Part model, mm, in its own coordinate system. A direction names the side the tool comes from. Round coordinates to 2 decimals unless told otherwise and drop trailing zeros. Write each loop counter-clockwise with the first axis right and the second up, starting at its lowest first coordinate (ties: lowest second). Pieces come first, ordered by that corner, then holes. Notation, with made-up numbers: M 45,35.5 L 87,35.5 A19 ccw 87,59.5 Z; hole C 44,-20 d9. An arc over 180 degrees is marked long. Use a Markdown table: item, result. Add a question column.
1) Which spindle directions (+Z, -Z, +X, -X, +Y, -Y) get a long thin tool onto all of the face, cutting with end or side? Do faces 1 (the face through (72.697, -22.893, 17.517)), 2 (the face through (-50.3, 15.4, 155.245)). Say none if no direction does.
2) Slice it at A-A on z = 73. Write the cut outline in (x, y), plus the area to 3 significant figures.
3) Wall check: probe 1 along X at (y, z) = (0, 77); probe 2 along Z at (x, y) = (-29, -63.5). Give the ranges that are in metal, low to high.
4) Drop flat-ended pins along their axis: P1, Ø8, axis at x = 22, y = 6.5, coming from the +Z side; P2, Ø4, axis at x = -3, z = 56, coming from the -Y side; P3, Ø10, axis at x = 4.5, z = 87.5, coming from the +Y side. Give the stop position or say it passes through.
5) Two-plate mould, pull along Z, no slides. Class faces 3 (the face through (-37.002, 28.372, 70.543)), 4 (the face through (35, -18, 0)), 5 (the face through (36.432, 70.045, 128.311)): released by +Z, released by -Z, zero draft, split by the parting line, or undercut.
6) Slice it at B-B on z = 90. Write the cut outline in (x, y).
```python
from build123d import *

# Parameters (mm, degrees)
F3_R = 5


# Not quite as in the source:
# - a feature of the source that left no trace in its solid (it failed there, or was rolled back) is left out


with BuildPart() as f2:
    # F0 (on Front) → F2 (revolve)
    with BuildSketch(Plane.XZ):
        with BuildLine():
            Line((38.9296258549, 0), (76.2161314487, 0))
            Line((76.2161314487, 0), (76.2161314487, 34.5504507422))
            ThreePointArc((76.2161314487, 34.5504507422), (55.3522757176, 42.613287739), (46.6280132532, 63.2093325257))
            Line((46.6280132532, 63.2093325257), (46.6280132532, 77.6744805479))
            ThreePointArc((46.6280132532, 77.6744805479), (56.3893375618, 99.0839330453), (78.9535716176, 105.7550236583))
            Line((78.9535716176, 105.7550236583), (78.9535716176, 155.2447585142))
            Line((78.9535716176, 155.2447585142), (46.4198933914, 155.2447585142))
            ThreePointArc((46.4198933914, 155.2447585142), (40.8771418071, 117.3123958387), (11.5445833653, 92.6306769252))
            Line((11.5445833653, 92.6306769252), (11.5445833653, 54.7694249827))
            ThreePointArc((11.5445833653, 54.7694249827), (32.356898751, 30.9446524602), (38.9296258549, 0))
        make_face()
    revolve(axis=Axis((0, 0, 66.4308094728), (0, 0, -1)))

    # F3
    f3_edges = [f2.edges().sort_by_distance(p)[0] for p in [
        (-78.953572, 0, 155.244759),
        (-46.419893, 0, 155.244759),
    ]]
    fillet(f3_edges, radius=F3_R)


solid = f2.part
```
Entries:
| question | item | result |
|---|---|---|
| 1 | face 1 | -Z |
| 1 | face 2 | +Z, +X, -X, +Y, -Y |
| 2 | outline | C 0,0 d93.26; hole C 0,0 d23.09 |
| 2 | area | 6,410 mm^2 |
| 3 | probe 1 | x = -46.63 to -11.54, 11.54 to 46.63 |
| 3 | probe 2 | z = 0 to 35.07, 105.56 to 155.24 |
| 4 | P1 | stops at z = 101.03 |
| 4 | P2 | stops at y = -48.06 |
| 4 | P3 | stops at y = 50.64 |
| 5 | face 3 | undercut |
| 5 | face 4 | released by -Z |
| 5 | face 5 | zero draft |
| 6 | outline | C 0,0 d98.89; hole C 0,0 d23.09 |
